Can you work these out from the drawing? Everything is in mm from the part's minimum corner. A direction names the side the tool comes from. Round coordinates to 2 decimals unless told otherwise and drop trailing zeros. Order: outer loops, then holes, each group sorted by start corner. A loop starts at its lowest first (then second) coordinate and runs counter-clockwise, first axis right, second up. Notation, with made-up numbers: (-22.5, 9) - (9.5, 9) arc R23 ccw to (9.5, 24) - close; hole circle Ø9 at (-34, 42). An arc over 180 degrees is marked (long way). Answer as a JSON object with one key per item and string values.
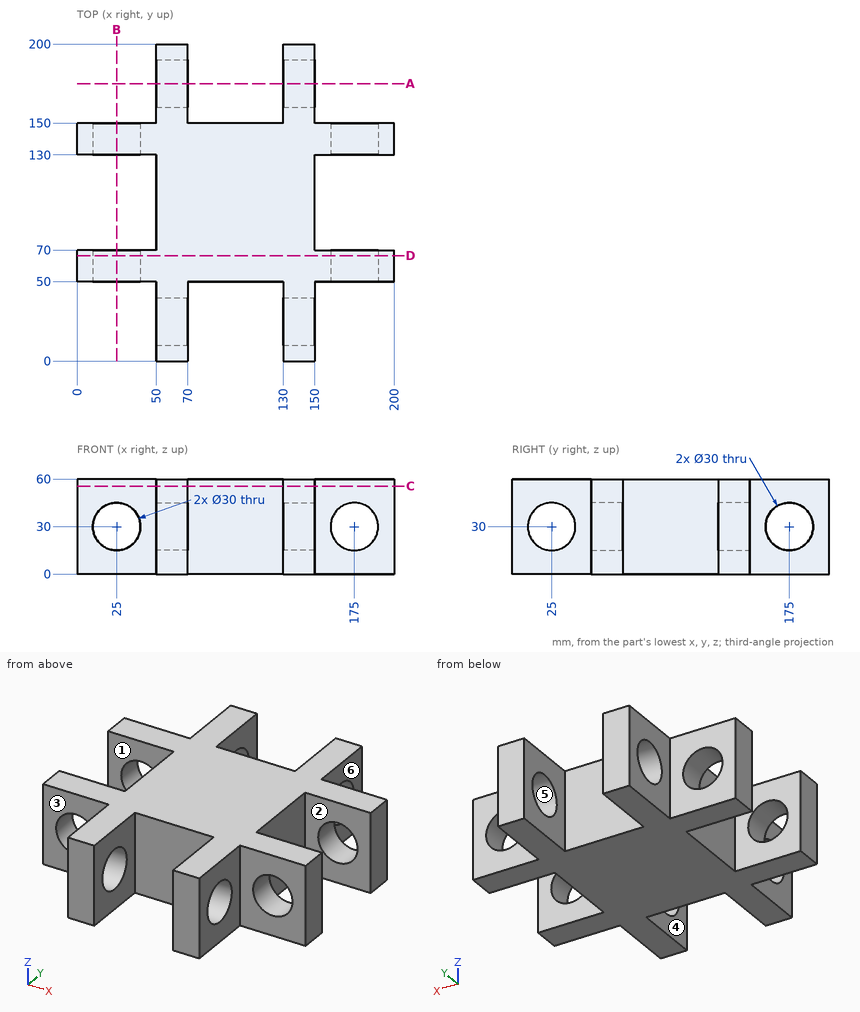
1. If I drill on L1, parallel to Y at x = 41.5, z = 50.5; L2, parallel to Z at x = 25, y = 65.25, over which ranges is the centre line in solid material (lowest first)? Write a range as [from, to].
Responses:
{"L1": "[50, 70], [130, 150]", "L2": "[0, 15], [45, 60]"}
2. Imagine slicing it at A-A (y = 175). List the corners of the cut face in (x, z) for me.
Responses:
{"outline": "(50, 0) - (70, 0) - (70, 15) - (50, 15) - close; (50, 45) - (70, 45) - (70, 60) - (50, 60) - close; (130, 0) - (150, 0) - (150, 15) - (130, 15) - close; (130, 45) - (150, 45) - (150, 60) - (130, 60) - close"}
3. Imagine slicing it at D-D (y = 66.5). List the corners of the cut face in (x, z) for me, plus the area to 3 significant figures.
Responses:
{"outline": "(0, 0) - (200, 0) - (200, 60) - (0, 60) - close; hole circle Ø30 at (25, 30); hole circle Ø30 at (175, 30)", "area": "10,600 mm2"}
4. Imagine slicing it at C-C (z = 55.5). List the corners of the cut face in (x, y) for me.
Responses:
{"outline": "(0, 50) - (50, 50) - (50, 0) - (70, 0) - (70, 50) - (130, 50) - (130, 0) - (150, 0) - (150, 50) - (200, 50) - (200, 70) - (150, 70) - (150, 130) - (200, 130) - (200, 150) - (150, 150) - (150, 200) - (130, 200) - (130, 150) - (70, 150) - (70, 200) - (50, 200) - (50, 150) - (0, 150) - (0, 130) - (50, 130) - (50, 70) - (0, 70) - close"}
5. For P1, Ø25, axis at x = 14, z = 44, coming from the +Y side; P2, Ø2, axis at y = 170, z = 44.5, coming from the +X side; P3, Ø2, axis at y = 83, z = 46.5, coming from the -X side, each with a flat end and sliding along its axis, tell me the tip position at first contact or that it passes through.
Responses:
{"P1": "y = 150", "P2": "x = 150", "P3": "x = 50"}
6. Thinking about a two-plate mould opening in X: for the marked faces 4, 5 and 6, which applies, pulls with the +X half, pulls with the -X half, needs draft (parallel to the pull), parting line crosses it, or undercut?
Responses:
{"face 4": "undercut", "face 5": "needs draft", "face 6": "pulls with the +X half"}
7. For the marked faces 1, 2 and 3, which set-ups out of +Z, -Z, +X, -X, +Y, -Y let a thin tool reach every point of the face, with its end or its side?
Responses:
{"face 1": "+Z, -Z, -X", "face 2": "+Z, -Z, +X", "face 3": "+Z, -Z, -X, -Y"}
